```python
from build123d import *

# Parameters (mm, degrees)
SKETCH1_W           = 203.2
SKETCH1_H           = 241.3
BOSS_EXTRUDE1_DEPTH = 6.35
SKETCH2_W           = 6.35
SKETCH2_H           = 25.4
SKETCH2_H_2         = 12.7
CUT_EXTRUDE2_DEPTH  = 7.62


with BuildPart() as part:
    # Sketch1 → Boss-Extrude1 (new body)
    with BuildSketch(Plane.XY):
        with Locations((-101.068226601, -2.674507389)):
            Rectangle(SKETCH1_W, SKETCH1_H)
    extrude(amount=BOSS_EXTRUDE1_DEPTH)

    # Sketch2 → Cut-Extrude2 (cut)
    with BuildSketch(Plane.XY.offset(6.35)):
        with Locations((-199.493226601, -85.224507389)):
            Rectangle(SKETCH2_W, SKETCH2_H)
        with Locations((-199.493226601, -34.424507389)):
            Rectangle(SKETCH2_W, SKETCH2_H)
        with Locations((-199.493226601, 16.375492611)):
            Rectangle(SKETCH2_W, SKETCH2_H)
        with Locations((-199.493226601, 67.175492611)):
            Rectangle(SKETCH2_W, SKETCH2_H)
        with Locations((-199.493226601, 111.625492611)):
            Rectangle(SKETCH2_W, SKETCH2_H_2)
        with Locations((-2.202282379, -85.224507389)):
            Rectangle(SKETCH2_W, SKETCH2_H)
        with Locations((-2.202282379, -34.424507389)):
            Rectangle(SKETCH2_W, SKETCH2_H)
        with Locations((-2.202282379, 16.208154802)):
            Rectangle(SKETCH2_W, SKETCH2_H)
        with Locations((-2.202282379, 67.008154802)):
            Rectangle(SKETCH2_W, SKETCH2_H)
        with Locations((-2.202282379, 111.458154802)):
            Rectangle(SKETCH2_W, SKETCH2_H_2)
    extrude(amount=-CUT_EXTRUDE2_DEPTH, mode=Mode.SUBTRACT)


solid = part.part
```
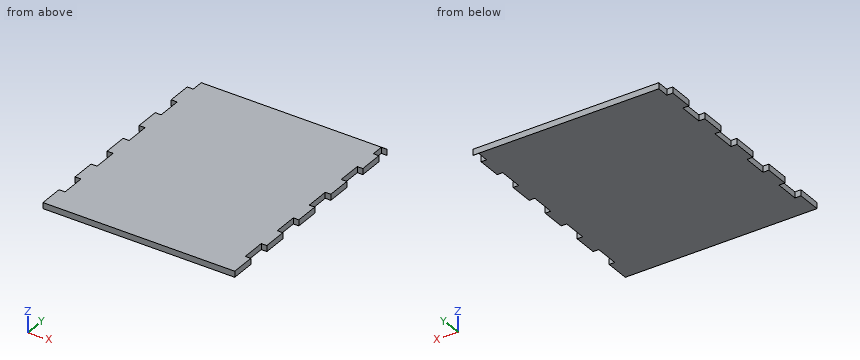
Could you check a few things on this model? Use its own coordinates, in mm. Give positions to 0.01 mm unless a question says otherwise; leave off trailing zeros. Write each loop counter-clockwise with the first axis right and the second up, starting at its lowest first coordinate (ties: lowest second). Pieces come first, ordered by that corner, then holes. Notation, with made-up numbers: (6, 66) - (28, 66) arc R27 cw to (28, 91) - close; hole circle Ø5 at (46, 1). An arc over 180 degrees is marked (long way). One line per item, written item: value. Start each with the question number.
Item 1: I'm going to push flat-ended pins straight in: pin 1 (3 mm diameter, centred on x = -199, z = 3.5, fed in from +Y); pin 2 (1.9 mm diameter, centred on y = -89, z = 2.5, fed in from +X). Where does each tip first touch, or does it pass through?
Item 2: Imagine slicing it at A-A, the plane y = 20. List the corners of the cut face in (x, z) for me, and give its area (3 significant figures).
Item 3: Please list where this line runs through material, in increasing order: line 1 (X direction, y = -25.5, z = 3.75). Write a range as from..to.
Geometry says:
1. pin 1: y = 105.28
1. pin 2: x = -5.38
2. outline: (-196.32, 0) - (-5.38, 0) - (-5.38, 6.35) - (-196.32, 6.35) - close
2. area: 1,210 mm^2
3. line 1: -196.32..-5.38
